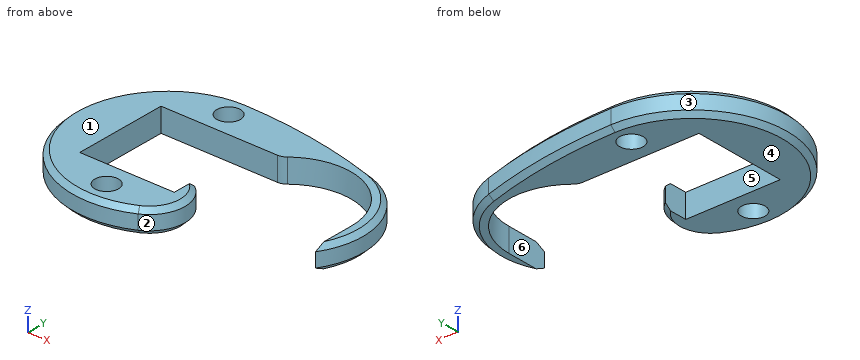
from build123d import *

# Parameters (mm, degrees)
BOSS_EXTRUDE1_DEPTH     = 3.175
FILLET1_R               = 3.175
SKETCH2_R               = 3.175
CUT_EXTRUDE1_DEPTH      = 1
CUT_EXTRUDE1_DEPTH_BACK = 7.35
CHAMFER1_SIZE           = 1.27


with BuildPart() as part:
    # Sketch1 → Boss-Extrude1 (new body, symmetric)
    with BuildSketch(Plane.XY):
        with BuildLine():
            Line((-19.05, -12.7), (-44.45, -12.7))
            Line((-44.45, -12.7), (-44.45, 12.7))
            Line((-44.45, 12.7), (-11.985362166, 12.7))
            ThreePointArc((-11.985362166, 12.7), (6.915364033, 16.034857235), (17.4625, 0))
            Line((17.4625, 0), (17.4625, -10.998522628))
            ThreePointArc((17.4625, -10.998522628), (19.34076991, 7.200071217), (6.019270833, 19.740181987))
            ThreePointArc((6.019270833, 19.740181987), (-12.632886304, 23.959177626), (-31.701893939, 25.399954445))
            ThreePointArc((-31.701893939, 25.399954445), (-56.451545619, -5.915542582), (-20.201381574, -22.622763148))
            ThreePointArc((-20.201381574, -22.622763148), (-15.030866787, -14.811488972), (-19.05, -6.35))
            Line((-19.05, -6.35), (-19.05, -12.7))
        make_face()
    extrude(amount=BOSS_EXTRUDE1_DEPTH, both=True)

    # Fillet1
    fillet1_edges = [part.edges().sort_by_distance(p)[0] for p in [
        (-11.985362166, 12.7, 0),
    ]]
    fillet(fillet1_edges, radius=FILLET1_R)

    # Sketch2 → Cut-Extrude1 (cut, two sides)
    with BuildSketch(Plane.XY.offset(3.175)) as cut_extrude1_sk:
        with Locations((-31.75, -19.05)):
            Circle(SKETCH2_R)
        with Locations((-31.75, 19.05)):
            Circle(SKETCH2_R)
    extrude(amount=CUT_EXTRUDE1_DEPTH, mode=Mode.SUBTRACT)
    extrude(cut_extrude1_sk.sketch, amount=-CUT_EXTRUDE1_DEPTH_BACK, mode=Mode.SUBTRACT)

    # Chamfer1
    chamfer1_edges = [part.edges().sort_by_distance(p)[0] for p in [
        (-15.030866787, -14.811488972, -3.175),
        (-56.451545619, -5.915542582, -3.175),
        (-12.632886304, 23.959177626, -3.175),
        (19.34076991, 7.200071217, -3.175),
        (19.34076991, 7.200071217, 3.175),
        (-12.632886304, 23.959177626, 3.175),
        (-56.451545619, -5.915542582, 3.175),
        (-15.030866787, -14.811488972, 3.175),
    ]]
    chamfer(chamfer1_edges, length=CHAMFER1_SIZE)


solid = part.part
Source: CAD feature listing. Evaluate the final solid. Frame: model axes, mm. Face numbers are marked on the shaded views. A direction names the side the tool comes from. Coordinates: 2 decimals unless noted, no trailing zeros.
Item 1: Cut plane A-A (z = -0.5). Count the separate pieces of the cut face and the enclosed holes in it, plus the area to 3 significant figures.
Output values:
separate pieces: 1
enclosed holes: 2
area: 1,260 mm2
Item 2: Pull-direction query (X, two-part tool) for the marked faces 1, 2 and 3; classes: pulls with the +X half, pulls with the -X half, needs draft (parallel to the pull), parting line crosses it, or undercut.
Output values:
face 1: needs draft
face 2: undercut
face 3: parting line crosses it
Item 3: Material intervals for line 1 (Y direction, x = -31.75, z = -0.25) (3 decimals); line 2 (Y direction, x = -31.75, z = -2) (3 decimals); line 3 (X direction, y = -10, z = -0.5), sorted ascending.
Output values:
line 1: y = -25.4 to -22.225, -15.875 to -12.7, 12.7 to 15.875, 22.225 to 25.4
line 2: y = -25.305 to -22.225, -15.875 to -12.7, 12.7 to 15.875, 22.225 to 25.305
line 3: x = -55.1 to -44.45, -19.05 to -15.95, 17.46 to 18.05
Item 4: First-contact query: P1, Ø1.5, axis at y = 11.5, z = 2, coming from the -X side; P2, Ø5, axis at x = -31.75, y = -19.05, coming from the -Z side; P3, Ø1.9, axis at x = -34.5, z = -1, coming from the -Y side; P4, Ø1.5, axis at y = 8.5, z = 1, coming from the -X side. Flat tips, straight axial feed; report the tip coordinate or a pass-through.
Output values:
P1: stops at x = -54.76
P2: passes through
P3: stops at y = -25.34
P4: stops at x = -55.94
Item 5: Set-up query: the marked faces 4, 5 and 6. Return all of +Z, -Z, +X, -X, +Y, -Y with unobstructed straight access to the full face (end or side cutting, diameter ignored); none if empty.
Output values:
face 4: -Z, +X, -X, +Y, -Y
face 5: +Z, -Z
face 6: +Z, -Z, -Y
